Geometry: final body of the model. Coordinates: model frame, mm. Face numbers are marked on the shaded views. A direction names the side the tool comes from. Give positions to 0.01 mm unless a question says otherwise; leave off trailing zeros. Write each loop counter-clockwise with the first axis right and the second up, starting at its lowest first coordinate (ties: lowest second). Pieces come first, ordered by that corner, then holes. Notation, with made-up numbers: (76.5, 8) - (80.5, 8) arc R24 cw to (80.5, 20) - close; hole circle Ø11 at (2.25, 40.5). An arc over 180 degrees is marked (long way). Return JSON: item names as keys, results as strings.
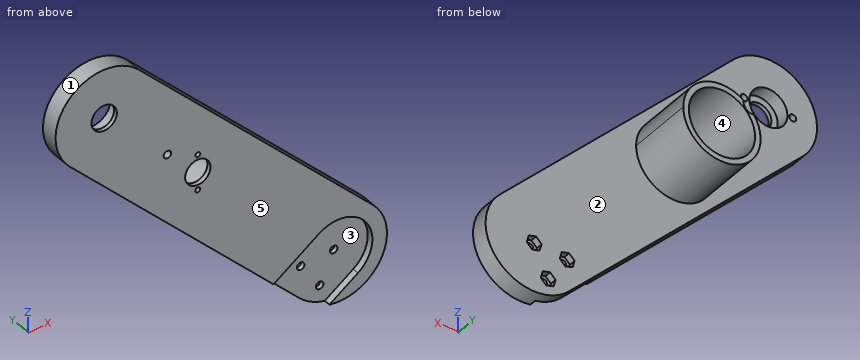
from build123d import *

# Parameters (mm, degrees)
BOSS_EXTRUDE1_DEPTH       = 8
BOSS_EXTRUDE3_START       = 8
SKETCH4_R                 = 15
BOSS_EXTRUDE3_DEPTH       = 30
CUT_EXTRUDE9_DEPTH        = 186.056233377
CUT_EXTRUDE9_DEPTH_BACK   = 186.056233377
SKETCH4_5_R               = 5.75
SKETCH4_5_R_2             = 1.1
SKETCH4_5_R_3             = 1.7
CUT_EXTRUDE5_START        = 8
SKETCH1_8_R               = 1.7
CUT_EXTRUDE5_DEPTH        = 3
CUT_EXTRUDE6_DEPTH        = 3
CUT_EXTRUDE11_START       = 1.8
SKETCH4_7_R               = 8.6
SKETCH4_7_R_2             = 5.75
SKETCH4_7_R_3             = 1.55
CUT_EXTRUDE11_DEPTH       = 6.2
CUT_EXTRUDE13_DEPTH       = 186.056233377
CUT_EXTRUDE13_DEPTH_BACK  = 186.056233377
SKETCH1_10_R              = 1.7
CUT_EXTRUDE14_START       = 2
CUT_EXTRUDE14_OUTLINE_R   = 15
CUT_EXTRUDE14_OUTLINE_R_2 = 1.1
CUT_EXTRUDE14_OUTLINE_R_3 = 5.75
CUT_EXTRUDE14_DEPTH       = 6


# Read off the part's stored shape, not the designer's step: Cut-Extrude14
with BuildPart() as part:
    # Sketch1 → Boss-Extrude1 (new body)
    with BuildSketch(Plane(origin=(0, 0, 0), x_dir=(1, 0, 0), z_dir=(0, 1, 0))):
        with BuildLine():
            Line((-15.556349186, 15.556349186), (90.509667992, 121.622366364))
            ThreePointArc((90.509667992, 121.622366364), (121.622366364, 121.622366364), (121.622366364, 90.509667992))
            Line((121.622366364, 90.509667992), (15.556349186, -15.556349186))
            ThreePointArc((15.556349186, -15.556349186), (-15.556349186, -15.556349186), (-15.556349186, 15.556349186))
        make_face()
    extrude(amount=BOSS_EXTRUDE1_DEPTH)

    # Sketch4 → Boss-Extrude3 (add)
    with BuildSketch(Plane(origin=(0, 0, 0), x_dir=(1, 0, 0), z_dir=(0, 1, 0)).offset(BOSS_EXTRUDE3_START)):
        with BuildLine():
            ThreePointArc((32.579864505, 27.95935453), (50.609789686, 26.957656252), (59.926406871, 42.426406871))
            ThreePointArc((59.926406871, 42.426406871), (37.274873894, 59.150990812), (27.95935453, 32.579864505))
            ThreePointArc((27.95935453, 32.579864505), (31.215238028, 31.696736244), (32.637824638, 28.637824638))
            ThreePointArc((32.637824638, 28.637824638), (32.623308264, 28.297353984), (32.579864505, 27.95935453))
        make_face()
        with Locations(Location((42.426406871, 42.426406871, 0), (0, 0, 270))):
            Circle(SKETCH4_R, mode=Mode.SUBTRACT)
    extrude(amount=BOSS_EXTRUDE3_DEPTH)

    # Sketch4<5> → Cut-Extrude9 (cut, two sides: drawn at the far end of the back side and taken through both)
    with BuildSketch(Plane(origin=(0, 0, 0), x_dir=(1, 0, 0), z_dir=(0, 1, 0)).offset(-CUT_EXTRUDE9_DEPTH_BACK)):
        with Locations(Location((0, 0, 0), (0, 0, 270))):
            Circle(SKETCH4_5_R)
        with Locations(Location((42.426406871, 42.426406871, 0), (0, 0, 270))):
            Circle(SKETCH4_5_R)
        with Locations(Location((42.426406871, 50.426406871, 0), (0, 0, 270))):
            Circle(SKETCH4_5_R_2)
        with Locations(Location((42.426406871, 34.426406871, 0), (0, 0, 270))):
            Circle(SKETCH4_5_R_2)
        with Locations(Location((28.637824638, 28.637824638, 0), (0, 0, 270))):
            Circle(SKETCH4_5_R_3)
    extrude(amount=CUT_EXTRUDE9_DEPTH + CUT_EXTRUDE9_DEPTH_BACK, mode=Mode.SUBTRACT)

    # Sketch1<8> → Cut-Extrude5 (cut)
    # profile 1 of 3: a face of its own
    with BuildSketch(Plane(origin=(0, 0, 0), x_dir=(1, 0, 0), z_dir=(0, 1, 0)).offset(CUT_EXTRUDE5_START)):
        Polygon((102.168353618, 117.21666144), (103.06492909, 120.562726655), (100.615439347, 123.012216398), (97.269374132, 122.115640925), (96.37279866, 118.769575711), (98.822288403, 116.320085968), align=None)
        with Locations(Location((99.718863875, 119.666151183, 0), (0, 0, 270))):
            Circle(SKETCH1_8_R, mode=Mode.SUBTRACT)
    # profile 2 of 3: a face of its own
    with BuildSketch(Plane(origin=(0, 0, 0), x_dir=(1, 0, 0), z_dir=(0, 1, 0)).offset(CUT_EXTRUDE5_START)):
        Polygon((88.665727587, 109.828360261), (87.769152115, 106.482295046), (90.218641857, 104.032805303), (93.564707072, 104.929380776), (94.461282545, 108.275445991), (92.011792802, 110.724935733), align=None)
        with Locations(Location((91.11521733, 107.378870518, 0), (0, 0, 270))):
            Circle(SKETCH1_8_R, mode=Mode.SUBTRACT)
    # profile 3 of 3: a face of its own
    with BuildSketch(Plane(origin=(0, 0, 0), x_dir=(1, 0, 0), z_dir=(0, 1, 0)).offset(CUT_EXTRUDE5_START)):
        Polygon((108.515506921, 103.616527435), (109.412082393, 106.96259265), (106.96259265, 109.412082393), (103.616527435, 108.515506921), (102.719951963, 105.169441706), (105.169441706, 102.719951963), align=None)
        with Locations(Location((106.066017178, 106.066017178, 0), (0, 0, 270))):
            Circle(SKETCH1_8_R, mode=Mode.SUBTRACT)
    extrude(amount=-CUT_EXTRUDE5_DEPTH, mode=Mode.SUBTRACT)

    # Sketch1<9> → Cut-Extrude6 (cut)
    with BuildSketch(Plane(origin=(0, 0, 0), x_dir=(1, 0, 0), z_dir=(0, 1, 0))):
        with BuildLine():
            Line((97.232940058, 93.451075696), (-12.006422067, 169.941300525))
            ThreePointArc((-12.006422067, 169.941300525), (-15.788286429, 191.389319127), (5.659732173, 195.171183489))
            Line((5.659732173, 195.171183489), (114.899094298, 118.68095866))
            ThreePointArc((114.899094298, 118.68095866), (118.68095866, 97.232940058), (97.232940058, 93.451075696))
        make_face()
    extrude(amount=CUT_EXTRUDE6_DEPTH, mode=Mode.SUBTRACT)

    # Sketch4<7> → Cut-Extrude11 (cut)
    # profile 1 of 3: a face of its own
    with BuildSketch(Plane(origin=(0, 0, 0), x_dir=(1, 0, 0), z_dir=(0, 1, 0)).offset(CUT_EXTRUDE11_START)):
        with Locations(Location((0, 0, 0), (0, 0, 270))):
            Circle(SKETCH4_7_R)
        with Locations(Location((0, 0, 0), (0, 0, 270))):
            Circle(SKETCH4_7_R_2, mode=Mode.SUBTRACT)
    # profile 2 of 3: a face of its own
    with BuildSketch(Plane(origin=(0, 0, 0), x_dir=(1, 0, 0), z_dir=(0, 1, 0)).offset(CUT_EXTRUDE11_START)):
        with Locations(Location((11, 0, 0), (0, 0, 270))):
            Circle(SKETCH4_7_R_3)
    # profile 3 of 3: a face of its own
    with BuildSketch(Plane(origin=(0, 0, 0), x_dir=(1, 0, 0), z_dir=(0, 1, 0)).offset(CUT_EXTRUDE11_START)):
        with Locations(Location((-11, 0, 0), (0, 0, 270))):
            Circle(SKETCH4_7_R_3)
    extrude(amount=CUT_EXTRUDE11_DEPTH, mode=Mode.SUBTRACT)

    # Sketch1<10> → Cut-Extrude13 (cut, two sides: drawn at the far end of the back side and taken through both)
    with BuildSketch(Plane(origin=(0, 0, 0), x_dir=(1, 0, 0), z_dir=(0, 1, 0)).offset(-CUT_EXTRUDE13_DEPTH_BACK)):
        with Locations(Location((99.718863875, 119.666151183, 0), (0, 0, 90))):
            Circle(SKETCH1_10_R)
        with Locations(Location((91.11521733, 107.378870518, 0), (0, 0, 90))):
            Circle(SKETCH1_10_R)
        with Locations(Location((106.066017178, 106.066017178, 0), (0, 0, 90))):
            Circle(SKETCH1_10_R)
    extrude(amount=CUT_EXTRUDE13_DEPTH + CUT_EXTRUDE13_DEPTH_BACK, mode=Mode.SUBTRACT)

    # Cut-Extrude14 outline → Cut-Extrude14 (cut)
    with BuildSketch(Plane(origin=(0, 0, 0), x_dir=(1, 0, 0), z_dir=(0, 1, 0)).offset(CUT_EXTRUDE14_START)):
        with Locations((42.426406871, 42.426406871)):
            Circle(CUT_EXTRUDE14_OUTLINE_R)
        with Locations((42.426406871, 34.426406871)):
            Circle(CUT_EXTRUDE14_OUTLINE_R_2, mode=Mode.SUBTRACT)
        with Locations((42.426406871, 42.426406871)):
            Circle(CUT_EXTRUDE14_OUTLINE_R_3, mode=Mode.SUBTRACT)
        with Locations((42.426406871, 50.426406871)):
            Circle(CUT_EXTRUDE14_OUTLINE_R_2, mode=Mode.SUBTRACT)
    extrude(amount=CUT_EXTRUDE14_DEPTH, mode=Mode.SUBTRACT)


solid = part.part
Q1. Mould query, pull axis X, two halves, no side actions, for the marked faces 1, 2 and 3. Classes: pulls with the +X half, pulls with the -X half, needs draft (parallel to the pull), parting line crosses it, or undercut.
Answer key:
{"face 1": "parting line crosses it", "face 2": "needs draft", "face 3": "undercut"}
Q2. Section query B-B, the plane x = 0. Return the cut outline in (y, z).
Answer key:
{"outline": "(0, -31.11) - (8, -31.11) - (8, -8.6) - (1.8, -8.6) - (1.8, -5.75) - (0, -5.75) - close; (0, 5.75) - (1.8, 5.75) - (1.8, 8.6) - (8, 8.6) - (8, 22) - (0, 22) - close"}
Q3. Section query A-A, the plane y = 19. Return the cut outline in (x, z), plus the area to 3 significant figures.
Answer key:
{"outline": "(27.96, -32.58) arc R17.5 ccw (long way) to (32.58, -27.96) arc R4 cw to start; hole circle Ø30 at (42.43, -42.43)", "area": "246 mm^2"}
Q4. Material intervals for probe 1 along Z at (x, y) = (42, 27); probe 2 along Y at (x, z) = (94, -100.5); probe 3 along Y at (x, z) = (119.5, -120.5), sorted ascending. Write a range as [from, to].
Answer key:
{"probe 1": "z = [-59.92, -57.42], [-27.43, -24.93]", "probe 2": "y = [3, 8]", "probe 3": "y = [0, 8]"}
Q5. Set-up query: the marked faces 4 and 5. Return all of +Z, -Z, +X, -X, +Y, -Y with unobstructed straight access to the full face (end or side cutting, diameter ignored); none if empty.
Answer key:
{"face 4": "+Y", "face 5": "+Z, -Z, +X, -X, -Y"}
Q6. Section query D-D, the plane x = 112. Return the cut outline in (y, z), plus the area to 3 significant figures.
Answer key:
{"outline": "(0, -127.25) - (8, -127.25) - (8, -80.89) - (0, -80.89) - (0, -91.86) - (3, -91.86) - (3, -120.71) - (0, -120.71) - close", "area": "284 mm^2"}
Q7. Section query C-C, the plane z = -45. Return the cut outline in (x, y).
Answer key:
{"outline": "(13.89, 0) - (37.28, 0) - (37.28, 2) - (27.65, 2) - (27.65, 38) - (25.12, 38) - (25.12, 8) - (13.89, 8) - close; (47.57, 0) - (76.11, 0) - (76.11, 8) - (59.74, 8) - (59.74, 38) - (57.2, 38) - (57.2, 2) - (47.57, 2) - close"}
Q8. Pin query (flat end, axial travel): P1, Ø3, axis at y = 31, z = -28.5, coming from the +X side; P2, Ø2.5, axis at x = 12, z = -0.5, coming from the +Y side; P3, Ø6, axis at x = 36, y = 14, coming from the +Z side; P4, Ø1, axis at x = 66, z = -81, coming from the -Y side. Return the tip coordinate at first contact, or that it passes through.
Answer key:
{"P1": "stops at x = 54.75", "P2": "stops at y = 8", "P3": "stops at z = -25.27", "P4": "stops at y = 0"}
